```python
from build123d import *

# Parameters (mm, degrees)
SKETCH_W        = 169
SKETCH_H        = 169
PAD_DEPTH       = 2
SKETCH002_W     = 20
SKETCH002_H     = 20
SKETCH002_W_2   = 22
SKETCH002_H_2   = 22
POCKET001_DEPTH = 2
SKETCH003_R     = 2
PAD001_DEPTH    = 2
SKETCH005_W     = 5
SKETCH005_H     = 5
PAD003_DEPTH    = 10
SKETCH007_W     = 5
SKETCH007_H     = 5
PAD004_DEPTH    = 10
SKETCH001_R     = 2.75
POCKET_DEPTH    = 2.001
SKETCH016_W     = 5
SKETCH016_H     = 5
PAD005_DEPTH    = 4
SKETCH017_W     = 2.5
SKETCH017_H     = 2
POCKET010_DEPTH = 5
SKETCH018_W     = 2.5
SKETCH018_H     = 2
POCKET011_DEPTH = 5
SKETCH019_W     = 2.5
SKETCH019_H     = 2
POCKET012_DEPTH = 2.5
SKETCH020_W     = 2.5
SKETCH020_H     = 2
POCKET013_DEPTH = 2.5
SKETCH021_W     = 2.5
SKETCH021_H     = 2.5
POCKET014_DEPTH = 5
SKETCH022_W     = 2.5
SKETCH022_H     = 2.5
POCKET015_DEPTH = 5
SKETCH023_W     = 2.5
SKETCH023_H     = 2.5
POCKET016_DEPTH = 5
SKETCH024_W     = 2.5
SKETCH024_H     = 2.5
POCKET017_DEPTH = 5
SKETCH025_W     = 2.5
SKETCH025_H     = 2.5
POCKET018_DEPTH = 5
SKETCH026_W     = 2.5
SKETCH026_H     = 2.5
POCKET019_DEPTH = 5
SKETCH027_W     = 2.5
SKETCH027_H     = 2.5
POCKET020_DEPTH = 5
SKETCH028_W     = 2.5
SKETCH028_H     = 2.5
POCKET021_DEPTH = 5


with BuildPart() as part:
    # Sketch (on DatumPlane) → Pad (new body)
    with BuildSketch(Plane.XY.offset(-2)):
        Rectangle(SKETCH_W, SKETCH_H)
    extrude(amount=PAD_DEPTH)

    # Sketch002 (on DatumPlane) → Pocket001 (cut)
    with BuildSketch(Plane.XY):
        with Locations((0, -65)):
            Rectangle(SKETCH002_W, SKETCH002_H)
        with Locations((0, 70)):
            Rectangle(SKETCH002_W_2, SKETCH002_H_2)
    extrude(amount=-POCKET001_DEPTH, mode=Mode.SUBTRACT)

    # Sketch003 (on DatumPlane) → Pad001 (join)
    with BuildSketch(Plane.XY):
        with Locations((-16, 72)):
            Circle(SKETCH003_R)
        with Locations((16, 72)):
            Circle(SKETCH003_R)
    extrude(amount=PAD001_DEPTH)

    # Sketch005 (on DatumPlane) → Pad003 (join)
    with BuildSketch(Plane.XY):
        with Locations((-12, 14.5)):
            Rectangle(SKETCH005_W, SKETCH005_H)
        with Locations((36.5, 14.5)):
            Rectangle(SKETCH005_W, SKETCH005_H)
        with Locations((-12, -15)):
            Rectangle(SKETCH005_W, SKETCH005_H)
        with Locations((36.5, -15)):
            Rectangle(SKETCH005_W, SKETCH005_H)
    extrude(amount=PAD003_DEPTH)

    # Sketch007 (on DatumPlane) → Pad004 (join)
    with BuildSketch(Plane.XY):
        with Locations((-73, -14)):
            Rectangle(SKETCH007_W, SKETCH007_H)
        with Locations((-30, -14)):
            Rectangle(SKETCH007_W, SKETCH007_H)
        with Locations((-73, -50)):
            Rectangle(SKETCH007_W, SKETCH007_H)
        with Locations((-30, -50)):
            Rectangle(SKETCH007_W, SKETCH007_H)
    extrude(amount=PAD004_DEPTH)

    # Sketch001 (on DatumPlane) → Pocket (cut, through all)
    with BuildSketch(Plane.XY):
        with Locations((75, 75)):
            Circle(SKETCH001_R)
        with Locations((75, -75)):
            Circle(SKETCH001_R)
        with Locations((-75, -75)):
            Circle(SKETCH001_R)
        with Locations((-75, 75)):
            Circle(SKETCH001_R)
    extrude(amount=-POCKET_DEPTH, mode=Mode.SUBTRACT)

    # Sketch016 (on DatumPlane) → Pad005 (join)
    with BuildSketch(Plane.XY):
        with Locations((-16, -30)):
            Rectangle(SKETCH016_W, SKETCH016_H)
        with Locations((16, -30)):
            Rectangle(SKETCH016_W, SKETCH016_H)
        with Locations((-16, -48)):
            Rectangle(SKETCH016_W, SKETCH016_H)
        with Locations((16, -48)):
            Rectangle(SKETCH016_W, SKETCH016_H)
    extrude(amount=PAD005_DEPTH)

    # Sketch017 (on Face36 of Pad005) → Pocket010 (cut)
    with BuildSketch(Plane.XZ.offset(32.5)):
        with Locations((-14.75, 1)):
            Rectangle(SKETCH017_W, SKETCH017_H)
    extrude(amount=-POCKET010_DEPTH, mode=Mode.SUBTRACT)

    # Sketch018 (on Face60 of Pocket010) → Pocket011 (cut)
    with BuildSketch(Plane.XZ.offset(32.5)):
        with Locations((14.75, 1)):
            Rectangle(SKETCH018_W, SKETCH018_H)
    extrude(amount=-POCKET011_DEPTH, mode=Mode.SUBTRACT)

    # Sketch019 (on Face35 of Pocket011) → Pocket012 (cut)
    with BuildSketch(Plane(origin=(0, -45.5, 0), x_dir=(-1, 0, 0), z_dir=(0, 1, 0))):
        with Locations((-14.75, 1)):
            Rectangle(SKETCH019_W, SKETCH019_H)
    extrude(amount=-POCKET012_DEPTH, mode=Mode.SUBTRACT)

    # Sketch020 (on Face38 of Pocket012) → Pocket013 (cut)
    with BuildSketch(Plane(origin=(0, -45.5, 0), x_dir=(-1, 0, 0), z_dir=(0, 1, 0))):
        with Locations((14.75, 1)):
            Rectangle(SKETCH020_W, SKETCH020_H)
    extrude(amount=-POCKET013_DEPTH, mode=Mode.SUBTRACT)

    # Sketch021 (on Face36 of Pocket013) → Pocket014 (cut)
    with BuildSketch(Plane.XY.offset(10)):
        with Locations((-71.75, -15.25)):
            Rectangle(SKETCH021_W, SKETCH021_H)
    extrude(amount=-POCKET014_DEPTH, mode=Mode.SUBTRACT)

    # Sketch022 (on Face87 of Pocket014) → Pocket015 (cut)
    with BuildSketch(Plane.XY.offset(10)):
        with Locations((-31.25, -15.25)):
            Rectangle(SKETCH022_W, SKETCH022_H)
    extrude(amount=-POCKET015_DEPTH, mode=Mode.SUBTRACT)

    # Sketch023 (on Face85 of Pocket015) → Pocket016 (cut)
    with BuildSketch(Plane.XY.offset(10)):
        with Locations((-71.75, -48.75)):
            Rectangle(SKETCH023_W, SKETCH023_H)
    extrude(amount=-POCKET016_DEPTH, mode=Mode.SUBTRACT)

    # Sketch024 (on Face73 of Pocket016) → Pocket017 (cut)
    with BuildSketch(Plane.XY.offset(10)):
        with Locations((-31.25, -48.75)):
            Rectangle(SKETCH024_W, SKETCH024_H)
    extrude(amount=-POCKET017_DEPTH, mode=Mode.SUBTRACT)

    # Sketch025 (on Face92 of Pocket017) → Pocket018 (cut)
    with BuildSketch(Plane.XY.offset(10)):
        with Locations((-10.75, 13.25)):
            Rectangle(SKETCH025_W, SKETCH025_H)
    extrude(amount=-POCKET018_DEPTH, mode=Mode.SUBTRACT)

    # Sketch026 (on Face87 of Pocket018) → Pocket019 (cut)
    with BuildSketch(Plane.XY.offset(10)):
        with Locations((35.25, 13.25)):
            Rectangle(SKETCH026_W, SKETCH026_H)
    extrude(amount=-POCKET019_DEPTH, mode=Mode.SUBTRACT)

    # Sketch027 (on Face85 of Pocket019) → Pocket020 (cut)
    with BuildSketch(Plane.XY.offset(10)):
        with Locations((-10.75, -13.75)):
            Rectangle(SKETCH027_W, SKETCH027_H)
    extrude(amount=-POCKET020_DEPTH, mode=Mode.SUBTRACT)

    # Sketch028 (on Face89 of Pocket020) → Pocket021 (cut)
    with BuildSketch(Plane.XY.offset(10)):
        with Locations((35.25, -13.75)):
            Rectangle(SKETCH028_W, SKETCH028_H)
    extrude(amount=-POCKET021_DEPTH, mode=Mode.SUBTRACT)


solid = part.part
```
For this review, take the finished solid that the model builds, in its own axes (mm). A direction names the side the tool comes from. Round coordinates to 2 decimals unless told otherwise and drop trailing zeros. Order: outer loops, then holes, each group sorted by start corner. A loop starts at its lowest first (then second) coordinate and runs counter-clockwise, first axis right, second up.
Q1. We need section A-A, the plane y = 62.5. Give the boundary of the cut face in (x, z).
Findings below:
outline: (-84.5, -2) - (-11, -2) - (-11, 0) - (-84.5, 0) - close; (11, -2) - (84.5, -2) - (84.5, 0) - (11, 0) - close
Q2. We need section C-C, the plane y = -22.5. Give the boundary of the cut face in (x, z), plus the area to 3 significant figures.
Findings below:
outline: (-84.5, -2) - (84.5, -2) - (84.5, 0) - (-84.5, 0) - close
area: 338 mm2
Q3. We need section B-B, the plane y = -67. Give the boundary of the cut face in (x, z), plus the area to 3 significant figures.
Findings below:
outline: (-84.5, -2) - (-10, -2) - (-10, 0) - (-84.5, 0) - close; (10, -2) - (84.5, -2) - (84.5, 0) - (10, 0) - close
area: 298 mm2
Q4. Machinability: for faces 1 (the flat face through (-70.5, -13, 4)), 2 (the flat face through (-13, 12, 4)), 3 (the flat face through (-73, -11.5, 5)), which of the approach directions +Z, -Z, +X, -X, +Y, -Y give a long, thin tool a straight path to every point of the face, cutting with its end or side? Answer none if there is none.
Findings below:
face 1: +Z, +Y, -Y
face 2: +Z, +X, -X
face 3: +Z, +X, -X, +Y
Q5. Mouldability with a two-part tool opening along X and no side actions: class faces 4 (the flat face through (-1, 1, -2)), 5 (the flat face through (13.5, -49, 2)), 6 (the flat face through (39, 14, 5)) as pulls with the +X half, pulls with the -X half, needs draft (parallel to the pull), parting line crosses it, or undercut.
Findings below:
face 4: needs draft
face 5: undercut
face 6: pulls with the +X half
Q6. Insertion check: P1, Ø5.5, axis at x = -74, z = 4.5, coming from the -Y side; P2, Ø6, axis at x = 19, y = 45, coming from the +Z side; P3, Ø1.6, axis at y = -30.5, z = 2.5, coming from the -X side; P4, Ø4, axis at x = -44, z = 2.5, coming from the +Y side. Each pin has a flat end and moves straight along its axis. Give the tip position at first contact, or say it passes through.
Findings below:
P1: stops at y = -52.5
P2: stops at z = 0
P3: stops at x = -18.5
P4: passes through
Q7. Wall thickness on line 1 (Y direction, x = 75, z = -0.35); line 2 (X direction, y = 13, z = 6.25); line 3 (Z direction, x = -40, y = 16): over which ranges is each line inside the solid? List them lowest first.
Findings below:
line 1: y = -84.5 to -77.75, -72.25 to 72.25, 77.75 to 84.5
line 2: x = -14.5 to -12, 36.5 to 39
line 3: z = -2 to 0
